Source: three-view drawing plus pictorial views. Frame: mm from the lowest corner of the part. A direction names the side the tool comes from. Give positions to 0.01 mm unless a question says otherwise; leave off trailing zeros. Loops run counter-clockwise (first coordinate to the right, second up) from the corner with the lowest first, then second, coordinate; pieces in that order, holes last. Notation, with made-up numbers: (75, 53) - (127, 53) arc R20 ccw to (127, 77) - close; hole circle Ø4 at (66.5, 77.25). An arc over 180 degrees is marked (long way). Answer as a JSON object with one key per item and string values. Group by question number.
(1) Access query for the marked faces 5 and 6. Directions: +Z, -Z, +X, -X, +Y, -Y. A direction counts if a zero-diameter tool reaches every point of the face in a straight line with its end or side. Return the directions, or none.
(2) Section query D-D (z = 13.25). Return loops of the section in (x, y).
(3) Section query C-C (z = 27.75). Return loops of the section in (x, y), plus the area to 3 significant figures.
(4) Material intervals for L1, parallel to Y at x = 25, z = 27.1; L2, parallel to Y at x = 25, z = 13; L3, parallel to Y at x = 24.5, z = 27.25 (1 decimal), sorted ascending.
(5) Mould query, pull axis X, two halves, no side actions, for the marked faces 1, 2, 3 and 4. Classes: +X half, -X half, draft (parallel to the pull), parting line (faces both ways), or undercut.
(6) Section query A-A (y = 10). Return loops of the section in (x, z), plus the area to 3 significant figures.
(7) Pin query (flat end, axial travel): P1, Ø6.5, axis at x = 10, y = 25, coming from the -Z side; P2, Ø10, axis at x = 38.5, z = 9, coming from the +Y side; P3, Ø12, axis at x = 29, z = 8, coming from the +Y side; P4, Ø12, axis at y = 5.5, z = 25.5, coming from the -X side. Return the tip coordinate at first contact, or that it passes through.
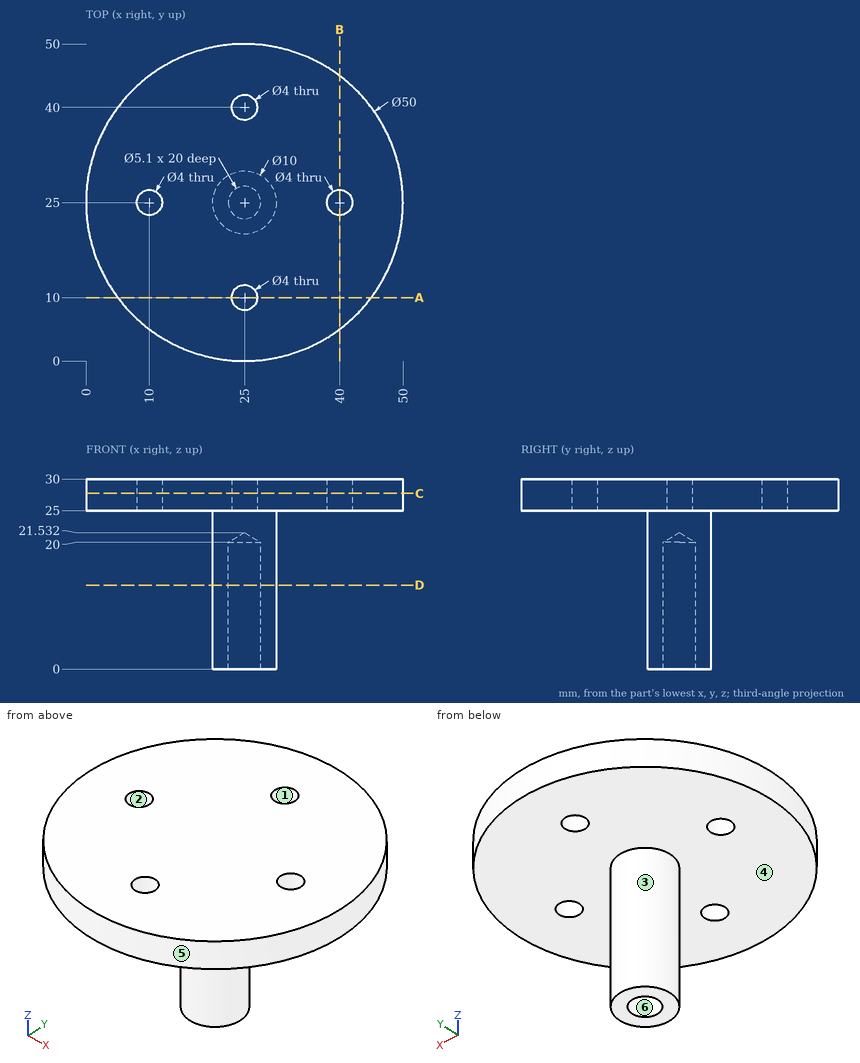
Recorded:
{
 "1": {"face 5": "+Z, -Z", "face 6": "-Z"},
 "2": {"outline": "circle Ø10 at (25, 25); hole circle Ø5.1 at (25, 25)"},
 "3": {"outline": "circle Ø50 at (25, 25); hole circle Ø4 at (10, 25); hole circle Ø4 at (25, 10); hole circle Ø4 at (25, 40); hole circle Ø4 at (40, 25)", "area": "1,910 mm^2"},
 "4": {"L1": "y = 0 to 8, 12 to 38, 42 to 50", "L2": "y = 20 to 22.45, 27.55 to 30", "L3": "y = 0 to 8.1, 11.9 to 38.1, 41.9 to 50"},
 "5": {"face 1": "undercut", "face 2": "undercut", "face 3": "parting line", "face 4": "draft"},
 "6": {"outline": "(5, 25) - (23, 25) - (23, 30) - (5, 30) - close; (27, 25) - (45, 25) - (45, 30) - (27, 30) - close", "area": "180 mm^2"},
 "7": {"P1": "stops at z = 25", "P2": "passes through", "P3": "stops at y = 30", "P4": "stops at x = 3.96"}
}
